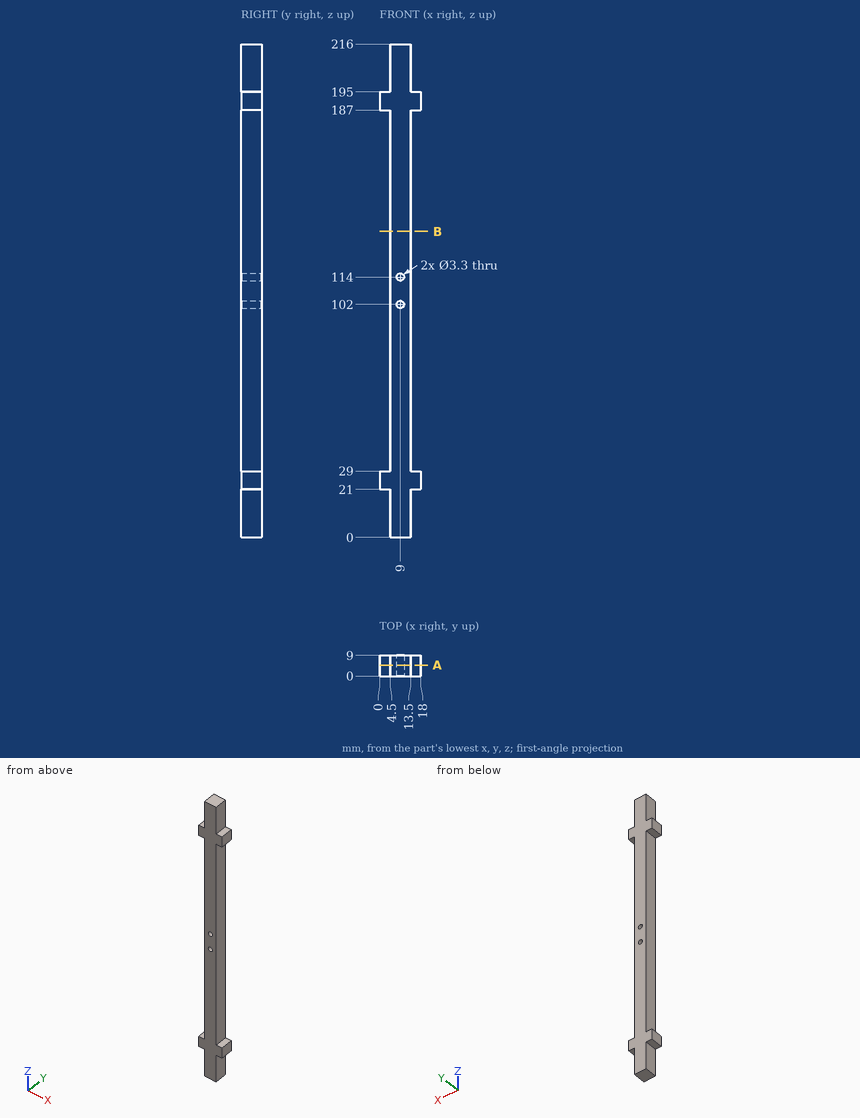
For this review, use the dimensioned drawing (mm, ordinates from the lowest corner) and the shaded views. Round coordinates to 2 decimals unless told otherwise and drop trailing zeros. Order: outer loops, then holes, each group sorted by start corner. A loop starts at its lowest first (then second) coordinate and runs counter-clockwise, first axis right, second up.
1) Clearance check with flat-ended pins moving along their axes: pin 1 Ø4.5 at (y, z) = (4, 14.5) entering from +X; pin 2 Ø4.5 at (y, z) = (4, 7.5) entering from -X; pin 3 Ø3.5 at (x, y) = (1.5, 6) entering from -Z. State where each tip first meets the part, or that it passes through.
The answers:
pin 1: stops at x = 13.5
pin 2: stops at x = 4.5
pin 3: stops at z = 21
2) Consider section B-B (z = 134). State the section outline as (x, y) points, plus the area to 3 significant figures.
The answers:
outline: (4.5, 0) - (13.5, 0) - (13.5, 9) - (4.5, 9) - close
area: 81.0 mm2
3) Consider section A-A (y = 4.75). State the section outline as (x, z) points.
The answers:
outline: (0, 21) - (4.5, 21) - (4.5, 0) - (13.5, 0) - (13.5, 21) - (18, 21) - (18, 29) - (13.5, 29) - (13.5, 187) - (18, 187) - (18, 195) - (13.5, 195) - (13.5, 216) - (4.5, 216) - (4.5, 195) - (0, 195) - (0, 187) - (4.5, 187) - (4.5, 29) - (0, 29) - close; hole circle Ø3.3 at (9, 102); hole circle Ø3.3 at (9, 114)
4) For L1, parallel to Z at x = 9, y = 3; L2, parallel to Z at x = 15, y = 7.25; L3, parallel to X at y = 2.5, z = 114, list the stretches that pass through material, from the lowest coordinate up.
The answers:
L1: z = 0 to 100.35, 103.65 to 112.35, 115.65 to 216
L2: z = 21 to 29, 187 to 195
L3: x = 4.5 to 7.35, 10.65 to 13.5
